```python
from build123d import *

# Parameters (mm, degrees)
F0_W     = 80
F0_H     = 81.325
F1_DEPTH = 0.75
F3_E1_W  = 27
F3_E1_H  = 1.5
F4_DEPTH = 7.5
F5_R     = 1
F7_W     = 7.6
F7_H     = 81.325
F8_DEPTH = 10


# Not quite as in the source:
# - two fillets or chamfers of one size are made in one step


with BuildPart() as f1:
    # F0 (on Top) → F1 (new body, symmetric)
    with BuildSketch(Plane.XY):
        Rectangle(F0_W, F0_H)
    extrude(amount=F1_DEPTH, both=True)

    # F3_E1 (on explicit) → F4 (join)
    with BuildSketch(Plane(origin=(-1.8, -40.6625, 0.75), x_dir=(1, 0, 0), z_dir=(0, 1, 0))):
        with Locations((13.5, 0.75)):
            Rectangle(F3_E1_W, F3_E1_H)
    extrude(amount=-F4_DEPTH)

    # F5
    f5_edges = [f1.edges().sort_by_distance(p)[0] for p in [
        (-1.8, -48.1625, 0),
        (25.2, -48.1625, 0),
    ]]
    fillet(f5_edges, radius=F5_R)

    # F7 (on face) → F8 (join)
    with BuildSketch(Plane.XY.offset(0.75)):
        with Locations((-36.2, 0)):
            Rectangle(F7_W, F7_H)
    extrude(amount=F8_DEPTH)


solid = f1.part
```
Check sheet for the modelled part. Datum: model origin and axes. Units: mm. A direction names the side the tool comes from. Round coordinates to 2 decimals unless told otherwise and drop trailing zeros. Order: outer loops, then holes, each group sorted by start corner. A loop starts at its lowest first (then second) coordinate and runs counter-clockwise, first axis right, second up.
1) Section check A-A (y = -24.5). Record the boundary of the cut face in (x, z).
2) Section check B-B (z = 6). Record the boundary of the cut face in (x, y).
3) Go/stop test with flat-tipped pins: pin 1 Ø21.5 at (x, y) = (16.5, 11) entering from +Z; pin 2 Ø1 at (y, z) = (27, 4.5) entering from +X; pin 3 Ø0.8 at (y, z) = (-44, 0) entering from +X. Record where each tip stops, or that it passes through.
4) Scan lines: line 1 (Y direction, x = -27, z = 0.5); line 2 (X direction, y = -29, z = 5.5); line 3 (Z direction, x = -22, y = 35). Record each from-to range of solid material in increasing order.
5) Section check C-C (x = 35). Record the boundary of the cut face in (y, z).
6) Tool access check on faces 1 (the flat face through (-29, -40.662, 0)), 2 (the flat face through (-15, 40.662, 0)), 3 (the flat face through (-32.4, -1, 6)). Record the directions out of +Z, -Z, +X, -X, +Y, -Y that give a thin tool (end or side, any length) a straight path to the whole face; none if there is none.
Result:
1. outline: (-40, -0.75) - (40, -0.75) - (40, 0.75) - (-32.4, 0.75) - (-32.4, 10.75) - (-40, 10.75) - close
2. outline: (-40, -40.66) - (-32.4, -40.66) - (-32.4, 40.66) - (-40, 40.66) - close
3. pin 1: stops at z = 0.75
3. pin 2: stops at x = -32.4
3. pin 3: stops at x = 25.2
4. line 1: y = -40.66 to 40.66
4. line 2: x = -40 to -32.4
4. line 3: z = -0.75 to 0.75
5. outline: (-40.66, -0.75) - (40.66, -0.75) - (40.66, 0.75) - (-40.66, 0.75) - close
6. face 1: +Z, -Z, -X, -Y
6. face 2: +Z, -Z, +X, -X, +Y
6. face 3: +Z, +X, +Y, -Y
